For this review, take the finished solid that the model builds, in its own axes (mm). A direction names the side the tool comes from. Give positions to 0.01 mm unless a question says otherwise; leave off trailing zeros. Write each loop counter-clockwise with the first axis right and the second up, starting at its lowest first coordinate (ties: lowest second). Pieces come first, ordered by that corner, then holes. Notation, with made-up numbers: M 63.25,29 L 104.25,29 A10 cw 104.25,33 Z; hole C -11,28.25 d1. An arc over 180 degrees is marked long. Answer as a JSON object with one key per item and string values. Group by question number.
```python
from build123d import *

# Parameters (mm, degrees)
SKETCH2_R           = 61.9125
SKETCH2_R_2         = 2.5
SKETCH2_R_3         = 52.3875
SKETCH2_R_4         = 4.5
SKETCH2_R_5         = 27.4955
SKETCH2_R_6         = 12.7
SKETCH2_R_7         = 3.3
BOSS_EXTRUDE1_DEPTH = 7.62
CUT_EXTRUDE1_DEPTH  = 997.881811459
FILLET2_R           = 12.7
CUT_EXTRUDE2_DEPTH  = 997.881811459
FILLET3_R           = 6.604


with BuildPart() as part:
    # Sketch2 → Boss-Extrude1 (new body)
    # profile 1 of 6: a face of its own
    with BuildSketch(Plane(origin=(0, 31.381947118, 0), x_dir=(1, 0, 0), z_dir=(0, 1, 0))):
        with Locations((-858.69104046, -110.005453999)):
            Circle(SKETCH2_R)
        with Locations((-864.664842136, -166.842380319)):
            Circle(SKETCH2_R_2, mode=Mode.SUBTRACT)
        with Locations((-820.450226307, -152.476180775)):
            Circle(SKETCH2_R_2, mode=Mode.SUBTRACT)
        with Locations((-801.54104046, -110.005453999)):
            Circle(SKETCH2_R_2, mode=Mode.SUBTRACT)
        with Locations((-816.220313684, -71.764639846)):
            Circle(SKETCH2_R_2, mode=Mode.SUBTRACT)
        with Locations((-858.69104046, -52.855453999)):
            Circle(SKETCH2_R_2, mode=Mode.SUBTRACT)
        with Locations((-904.926361688, -76.41352683)):
            Circle(SKETCH2_R_2, mode=Mode.SUBTRACT)
        with Locations((-915.52796678, -115.979255675)):
            Circle(SKETCH2_R_2, mode=Mode.SUBTRACT)
        with Locations((-901.161767236, -148.246268152)):
            Circle(SKETCH2_R_2, mode=Mode.SUBTRACT)
        with Locations((-858.69104046, -110.005453999)):
            Circle(SKETCH2_R_3, mode=Mode.SUBTRACT)
    # profile 2 of 6: a face of its own
    with BuildSketch(Plane(origin=(0, 31.381947118, 0), x_dir=(1, 0, 0), z_dir=(0, 1, 0))):
        with BuildLine():
            Line((-977.828766149, -19.064367123), (-913.231203194, -139.306107665))
            ThreePointArc((-913.231203194, -139.306107665), (-873.797989705, -49.964320259), (-796.77854046, -110.005453999))
            ThreePointArc((-796.77854046, -110.005453999), (-797.01050218, -115.359784371), (-797.704649202, -120.673993615))
            Line((-797.704649202, -120.673993615), (-732.205854251, -132.131902082))
            ThreePointArc((-732.205854251, -132.131902082), (-697.288937413, -95.264642324), (-649.722430089, -113.035779166))
            Line((-649.722430089, -113.035779166), (-727.765593148, -5.590386169))
            ThreePointArc((-727.765593148, -5.590386169), (-725.962377851, -9.130214457), (-725.34104046, -13.053976628))
            ThreePointArc((-725.34104046, -13.053976628), (-747.021296581, -22.034232749), (-738.04104046, -0.353976628))
            Line((-738.04104046, -0.353976628), (-966.64104046, -0.353976628))
            ThreePointArc((-966.64104046, -0.353976628), (-957.660784339, -4.073720507), (-953.94104046, -13.053976628))
            ThreePointArc((-953.94104046, -13.053976628), (-963.542179076, -25.370106626), (-977.828766149, -19.064367123))
        make_face()
    # profile 3 of 6: a face of its own
    with BuildSketch(Plane(origin=(0, 31.381947118, 0), x_dir=(1, 0, 0), z_dir=(0, 1, 0))):
        with BuildLine():
            ThreePointArc((-663.719686073, -177.370678379), (-662.142049476, -178.105218992), (-660.461885462, -177.651858179))
            ThreePointArc((-660.461885462, -177.651858179), (-688.572459971, -94.109699917), (-710.607035859, -179.455901191))
            ThreePointArc((-710.607035859, -179.455901191), (-708.047835111, -179.48984757), (-706.758334948, -177.278999281))
            Line((-706.758334948, -177.278999281), (-706.758334948, -176.701988839))
            ThreePointArc((-706.758334948, -176.701988839), (-700.258334948, -170.201988839), (-693.758334948, -176.701988839))
            Line((-693.758334948, -176.701988839), (-693.758334948, -183.274721629))
            ThreePointArc((-693.758334948, -183.274721629), (-693.101169654, -184.979577479), (-691.469725918, -185.802250576))
            ThreePointArc((-691.469725918, -185.802250576), (-686.919549358, -186.027976628), (-682.369372798, -185.802250576))
            ThreePointArc((-682.369372798, -185.802250576), (-680.737929062, -184.979577479), (-680.080763768, -183.274721629))
            Line((-680.080763768, -183.274721629), (-680.080763768, -176.701988839))
            ThreePointArc((-680.080763768, -176.701988839), (-676.068206079, -170.696771877), (-668.984569691, -172.105794761))
            Line((-668.984569691, -172.105794761), (-663.719686073, -177.370678379))
        make_face()
        with Locations((-686.919549358, -179.053976628)):
            Circle(SKETCH2_R_4, mode=Mode.SUBTRACT)
        with Locations((-661.85083258, -169.92970991)):
            Circle(SKETCH2_R_4, mode=Mode.SUBTRACT)
        with Locations((-648.51204699, -146.826255557)):
            Circle(SKETCH2_R_4, mode=Mode.SUBTRACT)
        with Locations((-653.14455861, -120.553976628)):
            Circle(SKETCH2_R_4, mode=Mode.SUBTRACT)
        with Locations((-673.580763768, -103.405964417)):
            Circle(SKETCH2_R_4, mode=Mode.SUBTRACT)
        with Locations((-700.258334948, -103.405964417)):
            Circle(SKETCH2_R_4, mode=Mode.SUBTRACT)
        with Locations((-720.694540106, -120.553976628)):
            Circle(SKETCH2_R_4, mode=Mode.SUBTRACT)
        with Locations((-725.327051725, -146.826255557)):
            Circle(SKETCH2_R_4, mode=Mode.SUBTRACT)
        with Locations((-711.988266136, -169.92970991)):
            Circle(SKETCH2_R_4, mode=Mode.SUBTRACT)
        with Locations((-686.919549358, -140.053976628)):
            Circle(SKETCH2_R_5, mode=Mode.SUBTRACT)
    # profile 4 of 6: a face of its own
    with BuildSketch(Plane(origin=(0, 31.381947118, 0), x_dir=(1, 0, 0), z_dir=(0, 1, 0))):
        with Locations((-966.64104046, -13.053976628)):
            Circle(SKETCH2_R_6)
        with Locations((-966.64104046, -13.053976628)):
            Circle(SKETCH2_R_7, mode=Mode.SUBTRACT)
    # profile 5 of 6: a face of its own
    with BuildSketch(Plane(origin=(0, 31.381947118, 0), x_dir=(1, 0, 0), z_dir=(0, 1, 0))):
        with Locations((-738.04104046, -13.053976628)):
            Circle(SKETCH2_R_6)
        with Locations((-738.04104046, -13.053976628)):
            Circle(SKETCH2_R_7, mode=Mode.SUBTRACT)
    # profile 6 of 6: a face of its own
    with BuildSketch(Plane(origin=(0, 31.381947118, 0), x_dir=(1, 0, 0), z_dir=(0, 1, 0))):
        with BuildLine():
            Line((-861.92593364, -171.83338557), (-709.563399524, -179.805130863))
            ThreePointArc((-709.563399524, -179.805130863), (-710.104359013, -179.687717863), (-710.607035859, -179.455901191))
            ThreePointArc((-710.607035859, -179.455901191), (-728.743420505, -159.142519743), (-732.205854251, -132.131902082))
            Line((-732.205854251, -132.131902082), (-797.704649202, -120.673993615))
            ThreePointArc((-797.704649202, -120.673993615), (-820.11475592, -158.430942405), (-861.92593364, -171.83338557))
        make_face()
    extrude(amount=BOSS_EXTRUDE1_DEPTH)

    # Sketch3 → Cut-Extrude1 (cut, through all)
    with BuildSketch(Plane.XZ.offset(-31.381947118)):
        with BuildLine():
            Line((-966.64104046, 0.353976628), (-738.04104046, 0.353976628))
            ThreePointArc((-738.04104046, 0.353976628), (-740.069201275, 0.516968863), (-742.04530312, 1.001761871))
            Line((-742.04530312, 1.001761871), (-853.43712543, 38.010902819))
            Line((-853.43712543, 38.010902819), (-962.564577542, 1.025990509))
            ThreePointArc((-962.564577542, 1.025990509), (-964.575298912, 0.523106273), (-966.64104046, 0.353976628))
        make_face()
    extrude(amount=-CUT_EXTRUDE1_DEPTH, mode=Mode.SUBTRACT)

    # Fillet2
    fillet2_edges = [part.edges().sort_by_distance(p)[0] for p in [
        (-853.43712543, 35.191947118, 38.010902819),
    ]]
    fillet(fillet2_edges, radius=FILLET2_R)

    # Sketch4 → Cut-Extrude2 (cut, through all)
    with BuildSketch(Plane.XZ.offset(-31.381947118)):
        with BuildLine():
            Line((-709.563399524, 179.805130863), (-709.298334948, 179.818999281))
            ThreePointArc((-709.298334948, 179.818999281), (-709.431048514, 179.815529807), (-709.563399524, 179.805130863))
        make_face()
        with BuildLine():
            Line((-926.258021859, 93.58986443), (-962.98962965, 25.217742455))
            ThreePointArc((-962.98962965, 25.217742455), (-956.946285575, 21.25773965), (-954.040776426, 14.642481046))
            Line((-954.040776426, 14.642481046), (-873.267054524, 42.017893591))
            ThreePointArc((-873.267054524, 42.017893591), (-907.186246099, 60.175908684), (-926.258021859, 93.58986443))
        make_face()
        with BuildLine():
            ThreePointArc((-750.650603562, 14.566893802), (-741.92637281, 25.145055675), (-728.673155688, 21.629099653))
            Line((-728.673155688, 21.629099653), (-686.683328555, 79.438308061))
            Line((-686.683328555, 79.438308061), (-798.984695976, 74.369503266))
            ThreePointArc((-798.984695976, 74.369503266), (-815.675199469, 55.375736994), (-838.053995618, 43.60604936))
            Line((-838.053995618, 43.60604936), (-750.650603562, 14.566893802))
        make_face()
        with BuildLine():
            ThreePointArc((-733.967803565, 114.387293709), (-740.490453219, 141.627220261), (-732.380486266, 168.437423414))
            Line((-732.380486266, 168.437423414), (-812.781759902, 164.230756215))
            Line((-812.781759902, 164.230756215), (-733.967803565, 114.387293709))
        make_face()
        with BuildLine():
            Line((-703.801263295, 86.293435405), (-799.833041569, 147.025779805))
            ThreePointArc((-799.833041569, 147.025779805), (-789.353275134, 115.205728597), (-794.969548727, 82.178487805))
            Line((-794.969548727, 82.178487805), (-703.801263295, 86.293435405))
        make_face()
    extrude(amount=-CUT_EXTRUDE2_DEPTH, mode=Mode.SUBTRACT)

    # Fillet3
    fillet3_edges = [part.edges().sort_by_distance(p)[0] for p in [
        (-873.267054524, 35.191947118, 42.017893591),
        (-954.040776426, 35.191947118, 14.642481046),
        (-962.98962965, 35.191947118, 25.217742455),
        (-926.258021859, 35.191947118, 93.58986443),
        (-732.380486266, 35.191947118, 168.437423414),
        (-733.967803565, 35.191947118, 114.387293709),
        (-812.781759902, 35.191947118, 164.230756215),
        (-799.833041569, 35.191947118, 147.025779805),
        (-703.801263295, 35.191947118, 86.293435405),
        (-794.969548727, 35.191947118, 82.178487805),
        (-838.053995618, 35.191947118, 43.60604936),
        (-798.984695976, 35.191947118, 74.369503266),
        (-686.683328555, 35.191947118, 79.438308061),
        (-728.673155688, 35.191947118, 21.629099653),
        (-750.650603562, 35.191947118, 14.566893802),
    ]]
    fillet(fillet3_edges, radius=FILLET3_R)


solid = part.part
```
Item 1: Consider section B-B (z = 44.5). Give the boundary of the cut face in (x, y).
Item 2: Insertion check: P1, Ø7, axis at x = -653.14, z = 120.55, coming from the -Y side; P2, Ø2, axis at y = 35, z = 181.5, coming from the -X side; P3, Ø0.6, axis at y = 36.5, z = 177, coming from the +X side; P4, Ø1.5, axis at x = -777.5, y = 34, coming from the -Z side. Each pin has a flat end and moves straight along its axis. Give the tip position at first contact, or say it passes through.
Item 3: Consider section C-C (x = -777). Give the boundary of the cut face in (y, z).
Item 4: Consider section A-A (x = -877). Give the boundary of the cut face in (y, z).
Item 5: To check wall thickness, follow probe 1 along Z at (x, y) = (-701, 38.5); probe 2 along X at (y, z) = (33.25, 66); probe 3 along Z at (x, y) = (-698, 35). State the ranges of each line that lie inside material, in increasing order.
Item 6: Draft analysis for pull direction X (two halves, no side actions). For faces 1 (the cylindrical face through (-798.13, 35.25, 160.28)), 2 (the flat face through (-798, 31.382, 93)), 3 (the cylindrical face through (-686.983, 35.139, 186.028)), state which applies: released by +X, released by -X, zero draft, split by the parting line, or undercut.
Item 7: Consider section D-D (y = 37). State how many separate pieces and enclosed holes the cut face has, plus the area to 3 significant figures.
Item 8: Machinability: for faces 4 (the cylindrical face through (-826.41, 35.25, 43.71)), 5 (the flat face through (-680.081, 35, 180)), 6 (the flat face through (-794.968, 35.139, 18.585)), which of the approach directions +Z, -Z, +X, -X, +Y, -Y give a long, thin tool a straight path to every point of the face, cutting with its end or side? Answer none if there is none.
Result set:
{
 "1": {"outline": "M -964.16,31.38 L -952.63,31.38 L -952.63,39 L -964.16,39 Z; M -887.12,31.38 L -826.46,31.38 L -826.46,39 L -887.12,39 Z; M -712.06,31.38 L -699.5,31.38 L -699.5,39 L -712.06,39 Z"},
 "2": {"P1": "passes through", "P2": "stops at x = -693.76", "P3": "stops at x = -659.16", "P4": "stops at z = 12.53"},
 "3": {"outline": "M 31.38,12.62 L 39,12.62 L 39,23.32 L 31.38,23.32 Z; M 31.38,75.36 L 39,75.36 L 39,82.99 L 31.38,82.99 Z; M 31.38,132.59 L 39,132.59 L 39,141.6 L 31.38,141.6 Z; M 31.38,166.1 L 39,166.1 L 39,176.28 L 31.38,176.28 Z"},
 "4": {"outline": "M 31.38,30.03 L 39,30.03 L 39,60.92 L 31.38,60.92 Z; M 31.38,159.09 L 39,159.09 L 39,169.15 L 31.38,169.15 Z"},
 "5": {"probe 1": "z = 42.44 to 59.73, 78.79 to 98.97, 107.84 to 116.44, 163.67 to 170.24", "probe 2": "x = -952.61 to -941.08, -912.53 to -887.12, -830.27 to -804.86, -696.44 to -683.89", "probe 3": "z = 46.57 to 63.86, 78.49 to 99.51, 107.3 to 114.89, 165.22 to 170.61"},
 "6": {"face 1": "undercut", "face 2": "zero draft", "face 3": "split by the parting line"},
 "7": {"separate pieces": "1", "enclosed holes": "25", "area": "18,000 mm^2"},
 "8": {"face 4": "+Y, -Y", "face 5": "+Z, +Y, -Y", "face 6": "-Z, +Y, -Y"}
}
